The model under review builds one solid part; all positions refer to its coordinate system, in mm. A direction names the side the tool comes from. Give positions to 0.01 mm unless a question says otherwise; leave off trailing zeros. Order: outer loops, then holes, each group sorted by start corner. A loop starts at its lowest first (then second) coordinate and runs counter-clockwise, first axis right, second up. Notation, with made-up numbers: (23, 63.25) - (81, 63.25) arc R20 cw to (81, 94.25) - close; hole circle Ø4 at (-37.75, 11). An arc over 180 degrees is marked (long way). Write item = value, one per line. Start each with the question number.
1. For P1, Ø6, axis at x = 18.5, y = -18, coming from the +Z side; P2, Ø22.5, axis at y = 3, z = 16.5, coming from the +X side; P3, Ø22.5, axis at x = -5.5, z = 18, coming from the -Y side, all flat-tipped, find the tip position at first contact; note any pin that passes through.
2. We need section C-C, the plane z = -3.5. Give the boundary of the cut face in (x, y).
3. We need section A-A, the plane x = 40.5. Give the boundary of the cut face in (y, z).
4. We need section D-D, the plane x = 16. Give the boundary of the cut face in (y, z).
5. Mouldability with a two-part tool opening along Y and no side actions: class faces 6 (the flat face through (4, 11, 28)), 7 (the flat face through (38, -8, -8)), 8 (the flat face through (23, 20, 11)) as pulls with the +Y half, pulls with the -Y half, needs draft (parallel to the pull), parting line crosses it, or undercut.
6. We need section B-B, the plane y = 12.5. Give the boundary of the cut face in (x, z).
7. Wall thickness on probe 1 along Y at (x, z) = (37, 2); probe 2 along X at (y, z) = (-17.5, 20); probe 3 along Z at (x, y) = (19.5, -29): over which ranges is each line inside the solid? List them lowest first.
8. Machinability: for faces 1 (the flat face through (-28, 11, 28)), 2 (the flat face through (-40, 7, 64)), 3 (the flat face through (38, 8, -8)), 4 (the flat face through (-12, -10, 11)), 5 (the flat face through (-11, -32, -2)), which of the approach directions +Z, -Z, +X, -X, +Y, -Y give a long, thin tool a straight path to every point of the face, cutting with its end or side? Answer none if there is none.
from build123d import *

# Parameters (mm, degrees)
SKETCH1_W               = 96
SKETCH1_H               = 64
BOSS_EXTRUDE1_DEPTH     = 16
BOSS_EXTRUDE2_DEPTH     = 16
SKETCH3_W               = 40
SKETCH3_H               = 28
BOSS_EXTRUDE3_DEPTH     = 42
BOSS_EXTRUDE4_DEPTH     = 12
CUT_EXTRUDE1_DEPTH      = 87.162636914
CUT_EXTRUDE1_DEPTH_BACK = 87.162636914
SKETCH6_R               = 12
CUT_EXTRUDE2_DEPTH      = 103.449987799


with BuildPart() as part:
    # Sketch1 → Boss-Extrude1 (new body)
    with BuildSketch(Plane.XY):
        Rectangle(SKETCH1_W, SKETCH1_H)
    extrude(amount=-BOSS_EXTRUDE1_DEPTH)

    # Sketch2 → Boss-Extrude2 (add)
    with BuildSketch(Plane.ZY.offset(48)):
        Polygon((0, 32), (64, 32), (64, -18.946257373), (34, -32), (0, -32), align=None)
    extrude(amount=-BOSS_EXTRUDE2_DEPTH)

    # Sketch3 → Boss-Extrude3 (add)
    with BuildSketch(Plane(origin=(0, 32, 0), x_dir=(1, 0, 0), z_dir=(0, 1, 0))):
        with Locations((-12, -14)):
            Rectangle(SKETCH3_W, SKETCH3_H)
    extrude(amount=-BOSS_EXTRUDE3_DEPTH)

    # Sketch4 → Boss-Extrude4 (add)
    with BuildSketch(Plane(origin=(0, 32, 0), x_dir=(1, 0, 0), z_dir=(0, 1, 0))):
        Polygon((8, -28), (48, 0), (8, 0), align=None)
    extrude(amount=-BOSS_EXTRUDE4_DEPTH)

    # Sketch5 → Cut-Extrude1 (cut, two sides: drawn at the far end of the back side and taken through both)
    with BuildSketch(Plane.XY.offset(-CUT_EXTRUDE1_DEPTH_BACK)):
        with BuildLine():
            Line((48, -8), (48, 8))
            Line((48, 8), (28, 8))
            ThreePointArc((28, 8), (20, 0), (28, -8))
            Line((28, -8), (48, -8))
        make_face()
    extrude(amount=CUT_EXTRUDE1_DEPTH + CUT_EXTRUDE1_DEPTH_BACK, mode=Mode.SUBTRACT)

    # Sketch6 → Cut-Extrude2 (cut, through all)
    with BuildSketch(Plane(origin=(0, 32, 0), x_dir=(1, 0, 0), z_dir=(0, 1, 0))):
        with Locations((-12, -28)):
            Circle(SKETCH6_R)
    extrude(amount=-CUT_EXTRUDE2_DEPTH, mode=Mode.SUBTRACT)


solid = part.part
Model answer:
q1.P1 = 0
q1.P2 = 8
q1.P3 = -10
q2.outline = (-48, -32) - (48, -32) - (48, -8) - (28, -8) arc R8 cw to (28, 8) - (48, 8) - (48, 32) - (-48, 32) - close
q3.outline = (-32, -16) - (-8, -16) - (-8, 0) - (-32, 0) - close; (8, -16) - (32, -16) - (32, 5.25) - (20, 5.25) - (20, 0) - (8, 0) - close
q4.outline = (-32, -16) - (32, -16) - (32, 22.4) - (20, 22.4) - (20, 0) - (-32, 0) - close
q5.face_6 = needs draft
q5.face_7 = undercut
q5.face_8 = pulls with the -Y half
q6.outline = (-48, -16) - (48, -16) - (48, 0) - (8, 0) - (8, 28) - (0, 28) arc R12 cw to (-24, 28) - (-32, 28) - (-32, 64) - (-48, 64) - close
q7.probe_1 = 20 to 32
q7.probe_2 = -48 to -32
q7.probe_3 = -16 to 0
q8.face_1 = +Z, +X, +Y, -Y
q8.face_2 = +Z, +X, -X, +Y, -Y
q8.face_3 = +Z, -Z, +X
q8.face_4 = +Z, +X, -Y
q8.face_5 = +Z, -Z, +X, -X, -Y
